```python
from build123d import *

# Parameters (mm, degrees)
ESQUISSE15_R        = 1.5
BOSS_EXTRU_15_DEPTH = 3


with BuildPart() as part:
    # Esquisse15 → Boss.-Extru.15 (new body)
    with BuildSketch(Plane.XY):
        with BuildLine():
            ThreePointArc((84.615566757, 77.214807715), (79.410356581, 79.056476896), (77.32447165, 73.944232535))
            add(Edge.make_bspline(
                [(77.145713615, 30.055195656), (79.080308516, 38.622687362), (81.66327099, 48.786134392), (79.931018502, 63.688726471), (79.143562251, 69.313820095), (77.32447165, 73.944232535)],
                knots=[0, 0, 0, 0, 0.576573495, 0.676573495, 1, 1, 1, 1], degree=3))
            ThreePointArc((77.145713615, 30.055195656), (80.218465063, 25.261002777), (84.971318589, 28.39731752))
            add(Edge.make_bspline(
                [(101.238857322, 62.671617625), (98.376312092, 59.555241307), (94.899619815, 55.416000824), (88.227335604, 44.717523156), (86.528624586, 36.263368643), (84.971318589, 28.39731752)],
                knots=[0, 0, 0, 0, 0.311641153, 0.411641153, 1, 1, 1, 1], degree=3))
            ThreePointArc((101.238857322, 62.671617625), (101.788339756, 67.322427703), (97.546599361, 69.307271211))
            add(Edge.make_bspline(
                [(84.615566757, 77.214807715), (85.76555462, 74.945262877), (87.284529762, 71.896675961), (92.709580096, 69.538935669), (95.692727353, 68.955151445), (97.546599361, 69.307271211)],
                knots=[0, 0, 0, 0, 0.456100215, 0.556100215, 1, 1, 1, 1], degree=3))
        make_face()
        with Locations((81.047477623, 75.406842025)):
            Circle(ESQUISSE15_R, mode=Mode.SUBTRACT)
        with Locations((98.293004791, 65.377528352)):
            Circle(ESQUISSE15_R, mode=Mode.SUBTRACT)
        with Locations((81.047477623, 29.17415217)):
            Circle(ESQUISSE15_R, mode=Mode.SUBTRACT)
    extrude(amount=BOSS_EXTRU_15_DEPTH)


solid = part.part
```
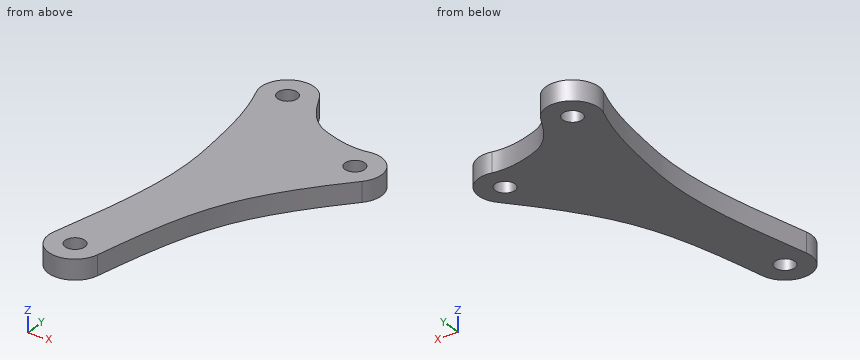
Geometry: final body of the model. Coordinates: model frame, mm. Round coordinates to 2 decimals unless told otherwise and drop trailing zeros. Answer in a Markdown table with one row per item. Add a question column.
(1) Contact query for flat-ended pins moving along their axis: pin 1 (1 mm diameter, centred on y = 53.5, z = 2, fed in from +X); pin 2 (1.5 mm diameter, centred on x = 84, z = 2.5, fed in from -Y). Output: stop coordinate, or through.
(2) Ray query, L1, parallel to Y at x = 81.5, z = 1.3; L2, parallel to Y at x = 97.5, z = 1.35; L3, parallel to Y at x = 99, z = 1.9. Return the intervals inside material, ascending.
(3) Cut plane A-A, the plane z = 1.65. Give the number of separate pieces and of enclosed holes in the cut face, then the cut area to 3 significant figures.
Established:
| question | item | result |
|---|---|---|
| 1 | pin 1 | x = 94.12 |
| 1 | pin 2 | y = 25.84 |
| 2 | L1 | 25.2 to 27.74, 30.6 to 73.98, 76.84 to 79.38 |
| 2 | L2 | 58.4 to 64.1, 66.65 to 69.3 |
| 2 | L3 | 60.17 to 64.05, 66.7 to 69.31 |
| 3 | separate pieces | 1 |
| 3 | enclosed holes | 3 |
| 3 | area | 616 mm² |
